Build history of the part. All positions in model axes, mm. Face numbers are marked on the shaded views. A direction names the side the tool comes from. Coordinates: 2 decimals unless noted, no trailing zeros. Order: outer loops, then holes, each group sorted by start corner. A loop starts at its lowest first (then second) coordinate and runs counter-clockwise, first axis right, second up. Notation, with made-up numbers: (2.5, 22.25) -> (30.5, 22.25) arc R23 ccw to (30.5, 34.25) -> close; hole circle Ø2 at (-16, -14). An arc over 180 degrees is marked (long way). Write each question's results on one line, items separated by ' | '.
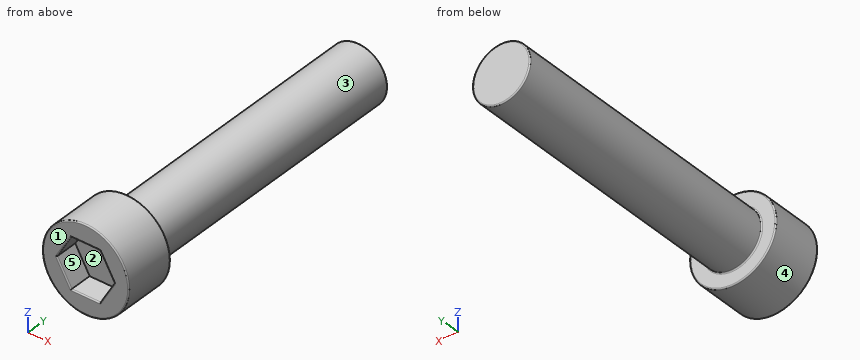
Solid Edge part; units mm, degrees
sketch "Sketch1" plane through (0, 0, 0) normal (0, -1, 0) x (1, 0, 0)
  circle A0 centre (0, 0) radius 3.75
extrude "Protrusion1" add sketch "Sketch1" along normal blind 4.5
sketch "Sketch2" plane through (0, 0, 0) normal (0, 1, 0) x (0, 0, -1)
  circle A0 centre (0, 0) radius 2.5
extrude "ExtrudedProtrusion_2" add sketch "Sketch2" along normal blind 25
sketch "Sketch3" plane through (0, -4.5, 0) normal (0, -1, 0) x (0, 0, 1)
  line L0 (-2.1651, 1.25) -> (-2.1651, -1.25)
  line L1 (-2.1651, -1.25) -> (0, -2.5)
  line L2 (0, -2.5) -> (2.1651, -1.25)
  line L3 (2.1651, -1.25) -> (2.1651, 1.25)
  line L4 (2.1651, 1.25) -> (0, 2.5)
  line L5 (0, 2.5) -> (-2.1651, 1.25)
extrude "ExtrudedCutout_1" cut sketch "Sketch3" against normal blind 2
fillet "Round_1" radius 0.1 10 edges at (-1.875, -4.5, 1.0825) (-1.875, -4.5, -1.0825) (0, -4.5, -2.1651) (1.875, -4.5, -1.0825) (1.875, -4.5, 1.0825) (0, -4.5, 2.1651) (-3.75, -4.5, 0) (-3.75, 0, 0) (0, 0, 2.5) (0, 25, 2.5)
Item 1: Slice it at A-A, the plane x = 0. List the corners of the cut face in (y, z), and give its area (3 significant figures).
Answer:
outline: (-4.5, -3.65) arc R0.1 ccw to (-4.4, -3.75) -> (-0.1, -3.75) arc R0.1 ccw to (0, -3.65) -> (0, -2.6) arc R0.1 cw to (0.1, -2.5) -> (24.9, -2.5) arc R0.1 ccw to (25, -2.4) -> (25, 2.4) arc R0.1 ccw to (24.9, 2.5) -> (0.1, 2.5) arc R0.1 cw to (0, 2.6) -> (0, 3.65) arc R0.1 ccw to (-0.1, 3.75) -> (-4.4, 3.75) arc R0.1 ccw to (-4.5, 3.65) -> (-4.5, 2.27) arc R0.1 ccw to (-4.4, 2.17) -> (-2.5, 2.17) -> (-2.5, -2.17) -> (-4.4, -2.17) arc R0.1 ccw to (-4.5, -2.27) -> close | area: 150 mm^2
Item 2: Pull direction X, two halves, no side cores. Call the marked faces 1, 2 and 3: released by +X, released by -X, zero draft, split by the parting line, or undercut.
Answer:
face 1: zero draft | face 2: undercut | face 3: split by the parting line
Item 3: Tool access for the marked faces 4 and 5: list every direction of +Z, -Z, +X, -X, +Y, -Y with a clear straight run to the whole face (end or side of a thin tool).
Answer:
face 4: +Y, -Y | face 5: -Y
Item 4: Slice it at B-B, the plane y = 1. List the corners of the cut face in (x, z), and give its area (3 significant figures).
Answer:
outline: circle Ø5 at (0, 0) | area: 19.6 mm^2
Item 5: Pin check, flat tips, straight feed: pin 1 (3 mm diameter, centred on x = -1, z = -2.5, fed in from +Y); pin 2 (4 mm diameter, centred on x = 2, y = 14.5, fed in from -Z); pin 3 (3 mm diameter, centred on x = 2.5, y = 15.5, fed in from -Z). Stop position of each tip, or through.
Answer:
pin 1: stops at y = 25 | pin 2: stops at z = -2.5 | pin 3: stops at z = -2.29
Item 6: Drill centre lines: line 1 (Z direction, x = 1.25, y = 17); line 2 (Y direction, x = 1.5, z = 1.25); line 3 (Y direction, x = 1.5, z = 3). Where is each one in solid material? Low to high. Write a range as from..to.
Answer:
line 1: z = -2.17..2.17 | line 2: y = -2.5..25 | line 3: y = -4.5..0
